The model under review builds one solid part; all positions refer to its coordinate system, in mm. Coordinates: 2 decimals unless noted, no trailing zeros. Order: outer loops, then holes, each group sorted by start corner. A loop starts at its lowest first (then second) coordinate and runs counter-clockwise, first axis right, second up. Notation, with made-up numbers: M -11.5,-25.75 L 13.5,-25.75 A21 ccw 13.5,-10.75 Z; hole C 17,77 d1. An arc over 180 degrees is marked long. Answer in a Markdown table with one row per item.
from build123d import *

# Parameters (mm, degrees)
F0_W     = 12.7
F0_H     = 76.2
F0_W_2   = 76.2
F0_H_2   = 12.7
F1_DEPTH = 12.7


with BuildPart() as f1:
    # F0 (on Top) → F1 (new body)
    with BuildSketch(Plane.XY):
        Polygon((-165.1, 101.6), (-203.2, 101.6), (-203.2, 38.1), (-190.5, 38.1), (-190.5, -38.1), (-203.2, -38.1), (-203.2, -101.6), (-165.1, -101.6), (-165.1, -88.9), (-88.9, -88.9), (-88.9, -101.6), (-38.1, -101.6), (-38.1, -88.9), (38.1, -88.9), (38.1, -101.6), (88.9, -101.6), (88.9, -88.9), (165.1, -88.9), (165.1, -101.6), (203.2, -101.6), (203.2, -38.1), (190.5, -38.1), (190.5, 38.1), (203.2, 38.1), (203.2, 101.6), (165.1, 101.6), (165.1, 88.9), (88.9, 88.9), (88.9, 101.6), (38.1, 101.6), (38.1, 88.9), (-38.1, 88.9), (-38.1, 101.6), (-88.9, 101.6), (-88.9, 88.9), (-165.1, 88.9), align=None)
        with Locations((-196.85, 0)):
            Rectangle(F0_W, F0_H)
        with Locations((-209.55, 0)):
            Rectangle(F0_W, F0_H)
        with Locations((0, 107.95)):
            Rectangle(F0_W_2, F0_H_2)
        with Locations((0, 95.25)):
            Rectangle(F0_W_2, F0_H_2)
        with Locations((0, -107.95)):
            Rectangle(F0_W_2, F0_H_2)
        with Locations((0, -95.25)):
            Rectangle(F0_W_2, F0_H_2)
        with Locations((196.85, 0)):
            Rectangle(F0_W, F0_H)
        with Locations((209.55, 0)):
            Rectangle(F0_W, F0_H)
        with Locations((-127, 107.95)):
            Rectangle(F0_W_2, F0_H_2)
        with Locations((-127, 95.25)):
            Rectangle(F0_W_2, F0_H_2)
        with Locations((127, 95.25)):
            Rectangle(F0_W_2, F0_H_2)
        with Locations((127, 107.95)):
            Rectangle(F0_W_2, F0_H_2)
        with Locations((127, -95.25)):
            Rectangle(F0_W_2, F0_H_2)
        with Locations((127, -107.95)):
            Rectangle(F0_W_2, F0_H_2)
        with Locations((-127, -95.25)):
            Rectangle(F0_W_2, F0_H_2)
        with Locations((-127, -107.95)):
            Rectangle(F0_W_2, F0_H_2)
    extrude(amount=F1_DEPTH)


solid = f1.part
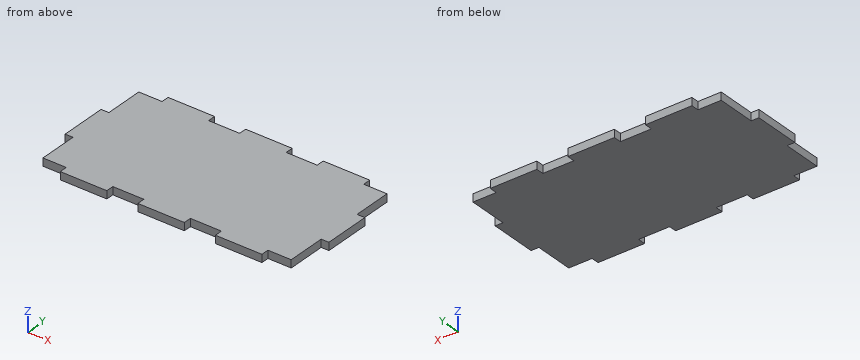
(1) Take a section at A-A (y = 90). Write out the cut boundary in (x, z).
Report:
| item | result |
|---|---|
| outline | M -203.2,0 L 203.2,0 L 203.2,12.7 L -203.2,12.7 Z |
(2) Take a section at B-B (x = -187). Write out the cut boundary in (y, z).
Report:
| item | result |
|---|---|
| outline | M -101.6,0 L 101.6,0 L 101.6,12.7 L -101.6,12.7 Z |
(3) Insertion check: P1, Ø1.5, axis at x = -47, z = 8.5, coming from the +Y side; P2, Ø6.5, axis at x = 54.5, z = 5, coming from the -Y side; P3, Ø4, axis at y = 108, z = 5.5, coming from the -X side. Each pin has a flat end and moves straight along its axis. Give the tip position at first contact, or say it passes through.
Report:
| item | result |
|---|---|
| P1 | y = 101.6 |
| P2 | y = -101.6 |
| P3 | x = -165.1 |
(4) To check wall thickness, follow line 1 (X direction, y = 61.5, z = 9.5); line 2 (Y direction, x = -48.5, z = 5). State the ranges of each line that lie inside material, in increasing order. Write a range as [from, to].
Report:
| item | result |
|---|---|
| line 1 | [-203.2, 203.2] |
| line 2 | [-101.6, 101.6] |
